Model file for the job. Use its own axes, mm. A direction names the side the tool comes from. Give positions to 0.01 mm unless a question says otherwise; leave off trailing zeros. Write each loop counter-clockwise with the first axis right and the second up, starting at its lowest first coordinate (ties: lowest second). Pieces come first, ordered by that corner, then holes.
```python
from build123d import *

# Parameters (mm, degrees)
SKETCH2_R           = 10
BOSS_EXTRUDE1_DEPTH = 40
SKETCH4_R           = 15
SKETCH4_R_2         = 4
BOSS_EXTRUDE2_DEPTH = 7.5


with BuildPart() as part:
    # Sketch2 → Boss-Extrude1 (new body)
    with BuildSketch(Plane.XY):
        Circle(SKETCH2_R)
    extrude(amount=BOSS_EXTRUDE1_DEPTH)

    # Sketch4 → Boss-Extrude2 (add, symmetric)
    with BuildSketch(Plane(origin=(0, 0, 0), x_dir=(1, 0, 0), z_dir=(0, 1, 0))):
        with Locations((-0.917156345, 14.971934552)):
            Circle(SKETCH4_R)
        with Locations((-0.917156345, 14.971934552)):
            Circle(SKETCH4_R_2, mode=Mode.SUBTRACT)
    extrude(amount=BOSS_EXTRUDE2_DEPTH, both=True)


solid = part.part
```
1. Slice it at C-C, the plane z = 29.5. Write the cut outline in (x, y).
Calculated:
outline: circle Ø20 at (0, 0)
2. Pin check, flat tips, straight feed: P1, Ø5, axis at x = 9.5, y = -3.5, coming from the -Z side; P2, Ø1.5, axis at y = -4, z = -12.5, coming from the +X side; P3, Ø5, axis at x = -12, z = -12.5, coming from the +Y side. Stop position of each tip, or through.
Calculated:
P1: stops at z = -27.71
P2: stops at x = 13.98
P3: stops at y = 7.5
3. Slice it at B-B, the plane y = -1.75. Write the cut outline in (x, z), and give its area (3 significant figures).
Calculated:
outline: (-9.85, 0) - (-1.83, 0) arc R15 ccw (long way) to (0, 0) - (9.85, 0) - (9.85, 40) - (-9.85, 40) - close; hole circle Ø8 at (-0.92, -14.97)
area: 1,440 mm2
4. Slice it at D-D, the plane y = 6.25. Write the cut outline in (x, z).
Calculated:
outline: (-7.81, 0) - (-1.83, 0) arc R15 ccw (long way) to (0, 0) - (7.81, 0) - (7.81, 40) - (-7.81, 40) - close; hole circle Ø8 at (-0.92, -14.97)
5. Pull direction X, two halves, no side cores. Call faces 1 (the flat face through (2, 7.5, -12)), 2 (the cylindrical face through (-1.438, -0.105, -18.938)), 3 (the cylindrical face through (-2.17, -9.76, 19.72)): +X half, -X half, draft (parallel to the pull), parting line (faces both ways), or undercut.
Calculated:
face 1: draft
face 2: undercut
face 3: parting line
6. Slice it at A-A, the plane x = 6.5. Write the cut outline in (y, z), and give its area (3 significant figures).
Calculated:
outline: (-7.6, 0) - (7.6, 0) - (7.6, 40) - (-7.6, 40) - close; (-7.5, -28.01) - (7.5, -28.01) - (7.5, -1.93) - (-7.5, -1.93) - close
area: 999 mm2
7. Probe probe 1 along X at (y, z) = (0.5, 1); probe 2 along Z at (x, y) = (-0.5, -8.5); probe 3 along Z at (x, y) = (7.75, 3). List the from-to ranges inside material, lowest first.
Calculated:
probe 1: x = -9.99 to 9.99
probe 2: z = 0 to 40
probe 3: z = -27.21 to -2.73, 0 to 40
8. Which spindle directions (+Z, -Z, +X, -X, +Y, -Y) get a long thin tool onto all of the face, cutting with end or side? Do faces 4 (the flat face through (2, -7.5, -12)), 5 (the flat face through (0, 0, 40)). Say none if no direction does.
Calculated:
face 4: -Z, +X, -X, -Y
face 5: +Z, +X, -X, +Y, -Y
